```python
from build123d import *

# Parameters (mm, degrees)
SKETCH_W           = 7
SKETCH_H           = 7
PAD_DEPTH          = 1.58
POCKET_DEPTH       = 0.5
SKETCH002_W        = 1.02
SKETCH002_H        = 1.02
PAD001_DEPTH       = 3.94
POLARPATTERN_COUNT = 4
SKETCH003_R        = 2.03
POCKET001_DEPTH    = 0.2
SKETCH004_R        = 0.635
PAD002_DEPTH       = 4.64
CHAMFER_SIZE       = 0.2
CHAMFER001_SIZE    = 0.1
CHAMFER002_SIZE    = 0.1


with BuildPart() as part:
    # Sketch → Pad (new body)
    with BuildSketch(Plane.XY):
        Rectangle(SKETCH_W, SKETCH_H)
    extrude(amount=PAD_DEPTH)

    # Sketch001 (on Face5 of Pad) → Pocket (cut)
    with BuildSketch(Plane(origin=(0, 0, 0), x_dir=(1, 0, 0), z_dir=(0, 0, -1))):
        Polygon((-3.5, 2.03), (-2.03, 2.03), (-2.03, 3.5), (2.03, 3.5), (2.03, 2.03), (3.5, 2.03), (3.5, -2.03), (2.03, -2.03), (2.03, -3.5), (-2.03, -3.5), (-2.03, -2.03), (-3.5, -2.03), align=None)
    extrude(amount=-POCKET_DEPTH, mode=Mode.SUBTRACT)

    # Sketch002 (on Face6 of Pocket) → Pad001 (join)
    with BuildSketch(Plane(origin=(0, 0, 0), x_dir=(1, 0, 0), z_dir=(0, 0, -1))):
        with Locations((-2.54, 2.54)):
            Rectangle(SKETCH002_W, SKETCH002_H)
    pad001 = extrude(amount=PAD001_DEPTH)

    # PolarPattern: Pad001 ×4 about axis
    polarpattern_axis = Axis((0, 0, 0), (0, 0, -1))
    for i in range(1, POLARPATTERN_COUNT):
        add(pad001.rotate(polarpattern_axis, i * 360 / POLARPATTERN_COUNT))

    # Sketch003 (on Face4 of PolarPattern) → Pocket001 (cut)
    with BuildSketch(Plane(origin=(0, 0, 0.5), x_dir=(1, 0, 0), z_dir=(0, 0, -1))):
        Circle(SKETCH003_R)
    extrude(amount=-POCKET001_DEPTH, mode=Mode.SUBTRACT)

    # Sketch004 (on Face33 of Pocket001) → Pad002 (join)
    with BuildSketch(Plane(origin=(0, 0, 0.7), x_dir=(1, 0, 0), z_dir=(0, 0, -1))):
        Circle(SKETCH004_R)
    extrude(amount=PAD002_DEPTH)

    # Chamfer
    chamfer_edges = [part.edges().sort_by_distance(p)[0] for p in [
        (-0.635, 0, -3.94),
    ]]
    chamfer(chamfer_edges, length=CHAMFER_SIZE)

    # Sketch005 → Revolution (revolve)
    with BuildSketch(Plane.XZ):
        Polygon((0, 1.58), (0, 12.26), (0.48, 12.26), (0.48, 15.46), (0.63, 15.46), (0.63, 14.96), (1.9, 14.96), (1.9, 15.58), (2.325, 15.58), (2.325, 17.58), (2.65, 17.58), (2.65, 2.766921), (3.095, 2.51), (3.095, 1.58), align=None)
    revolve(axis=Axis((0, 0, 0), (0, 0, 1)))

    # Chamfer001
    chamfer001_edges = [part.edges().sort_by_distance(p)[0] for p in [
        (-2.325, 0, 17.58),
        (-2.65, 0, 17.58),
    ]]
    chamfer(chamfer001_edges, length=CHAMFER001_SIZE)

    # Chamfer002
    chamfer002_edges = [part.edges().sort_by_distance(p)[0] for p in [
        (-0.48, 0, 15.46),
    ]]
    chamfer(chamfer002_edges, length=CHAMFER002_SIZE)

    # Sketch006 → Revolution001 (revolve)
    with BuildSketch(Plane.XZ):
        Polygon((2.65, 2.791559), (3.095, 3.04848), (3.095, 3.21612), (2.65, 3.473041), align=None)
        Polygon((2.65, 3.497679), (3.095, 3.7546), (3.095, 3.92224), (2.65, 4.179161), align=None)
        Polygon((2.65, 4.203799), (3.095, 4.46072), (3.095, 4.62836), (2.65, 4.885281), align=None)
        Polygon((2.65, 4.909919), (3.095, 5.16684), (3.095, 5.33448), (2.65, 5.591401), align=None)
        Polygon((2.65, 5.616039), (3.095, 5.87296), (3.095, 6.0406), (2.65, 6.297521), align=None)
        Polygon((2.65, 6.322159), (3.095, 6.57908), (3.095, 6.74672), (2.65, 7.003641), align=None)
        Polygon((2.65, 7.734399), (3.095, 7.99132), (3.095, 8.15896), (2.65, 8.415881), align=None)
        Polygon((2.65, 7.028279), (3.095, 7.2852), (3.095, 7.45284), (2.65, 7.709761), align=None)
        Polygon((2.65, 8.440519), (3.095, 8.69744), (3.095, 8.86508), (2.65, 9.122001), align=None)
        Polygon((2.65, 9.146639), (3.095, 9.40356), (3.095, 9.5712), (2.65, 9.828121), align=None)
        Polygon((2.65, 10.558879), (3.095, 10.8158), (3.095, 10.98344), (2.65, 11.240361), align=None)
        Polygon((2.65, 9.852759), (3.095, 10.10968), (3.095, 10.27732), (2.65, 10.534241), align=None)
        Polygon((2.65, 11.971119), (3.095, 12.22804), (3.095, 12.39568), (2.65, 12.652601), align=None)
        Polygon((2.65, 11.264999), (3.095, 11.52192), (3.095, 11.68956), (2.65, 11.946481), align=None)
        Polygon((2.65, 12.677239), (3.095, 12.93416), (3.095, 13.1018), (2.65, 13.358721), align=None)
        Polygon((2.65, 13.383359), (3.095, 13.64028), (3.095, 13.80792), (2.65, 14.064841), align=None)
        Polygon((2.65, 14.089479), (3.095, 14.3464), (3.095, 14.51404), (2.65, 14.770961), align=None)
        Polygon((2.65, 15.501719), (3.095, 15.75864), (3.095, 15.92628), (2.65, 16.183201), align=None)
        Polygon((2.65, 16.207839), (3.095, 16.46476), (3.095, 16.6324), (2.65, 16.889321), align=None)
        Polygon((2.65, 14.795599), (3.095, 15.05252), (3.095, 15.22016), (2.65, 15.477081), align=None)
    revolve(axis=Axis((0, 0, 0), (0, 0, 1)))


solid = part.part
```
Read the model definition and answer for the solid it produces. Units are mm, in the model's axes. A direction names the side the tool comes from. Give positions to 0.01 mm unless a question says otherwise; leave off trailing zeros.
Item 1: Find the intervals of material crossed by line 1 along Y through (x, z) = (0, 0.65) (3 decimals); line 2 along X through (y, z) = (-0.25, 15); line 3 along Z through (x, y) = (1, 2), in increasing order.
Item 2: For faces 1 (the flat face through (-2.5, -2.5, -3.94)), 2 (the flat face through (0, 0, 12.26)), 3 (the flat face through (3.05, 2.5, -1.9)), determine the directions among +Z, -Z, +X, -X, +Y, -Y from which every point of the face is accessible in a straight line to the end or side of a thin tool.
Item 3: Each of these flat-tipped pins is pushed along its axis until it touches: pin 1 Ø0.8 at (x, z) = (2.5, -3) entering from -Y; pin 2 Ø3 at (y, z) = (0, 10) entering from +X (3 decimals); pin 3 Ø0.5 at (x, z) = (2.5, -3) entering from +Y. Where does it stop, or does it pass through?
Taken from the geometry:
1. line 1: y = -3.5 to -2.03, -0.635 to 0.635, 2.03 to 3.5
1. line 2: x = -2.99 to -1.88, -0.58 to -0.41, 0.41 to 0.58, 1.88 to 2.99
1. line 3: z = 0.5 to 15.58
2. face 1: -Z, +X, -X, +Y, -Y
2. face 2: +Z
2. face 3: -Z, +X, +Y, -Y
3. pin 1: stops at y = -3.05
3. pin 2: stops at x = 3.095
3. pin 3: stops at y = 3.05
